The listing builds one solid part. Answer for the finished solid, in the listing's coordinates (mm). Face numbers are marked on the shaded views. Give positions to 0.01 mm unless a question says otherwise; leave off trailing zeros. Write each loop counter-clockwise with the first axis right and the second up, starting at its lowest first coordinate (ties: lowest second). Pieces come first, ordered by that corner, then holes.
```python
from build123d import *

# Parameters (mm, degrees)
SKETCH1_R           = 7
BOSS_EXTRUDE1_DEPTH = 1
SKETCH2_R           = 7
BOSS_EXTRUDE2_DEPTH = 4
SKETCH3_R           = 7.5
BOSS_EXTRUDE3_DEPTH = 1
SKETCH5_R           = 7
SKETCH7_R           = 7.5
BOSS_EXTRUDE4_DEPTH = 1
SKETCH8_R           = 7
BOSS_EXTRUDE5_DEPTH = 4
SKETCH9_R           = 7
BOSS_EXTRUDE6_DEPTH = 1
SKETCH11_R          = 6


with BuildPart() as part:
    # Sketch1 → Boss-Extrude1 (new body)
    with BuildSketch(Plane(origin=(0, 0, 0), x_dir=(1, 0, 0), z_dir=(0, 1, 0))):
        with Locations(Location((0, 0, 0), (0, 0, 270))):
            Circle(SKETCH1_R)
    extrude(amount=BOSS_EXTRUDE1_DEPTH)

    # Sketch2 → Boss-Extrude2 (add)
    with BuildSketch(Plane(origin=(0, 1, 0), x_dir=(1, 0, 0), z_dir=(0, 1, 0))):
        with Locations(Location((0, 0, 0), (0, 0, 270))):
            Circle(SKETCH2_R)
    extrude(amount=BOSS_EXTRUDE2_DEPTH)

    # Sketch3 → Boss-Extrude3 (add)
    with BuildSketch(Plane(origin=(0, 5, 0), x_dir=(1, 0, 0), z_dir=(0, 1, 0))):
        with Locations(Location((0, 0, 0), (0, 0, 270))):
            Circle(SKETCH3_R)
    extrude(amount=BOSS_EXTRUDE3_DEPTH)

    # Sweep1: sweep along a path in Sketch4
    with BuildLine(Plane.XY) as sweep1_path:
        ThreePointArc((0, 6), (6.443650814, 21.556349186), (22, 28))
    # Sketch5 → Sweep1 (sweep)
    with BuildSketch(Plane(origin=(0, 6, 0), x_dir=(1, 0, 0), z_dir=(0, 1, 0))):
        Circle(SKETCH5_R)
    sweep(path=sweep1_path.line)

    # Sketch7 → Boss-Extrude4 (add)
    with BuildSketch(Plane(origin=(22, 0, 0), x_dir=(0, 0, -1), z_dir=(1, 0, 0))):
        with Locations((0, 28)):
            Circle(SKETCH7_R)
    extrude(amount=BOSS_EXTRUDE4_DEPTH)

    # Sketch8 → Boss-Extrude5 (add)
    with BuildSketch(Plane(origin=(23, 0, 0), x_dir=(0, 0, -1), z_dir=(1, 0, 0))):
        with Locations((0, 28)):
            Circle(SKETCH8_R)
    extrude(amount=BOSS_EXTRUDE5_DEPTH)

    # Sketch9 → Boss-Extrude6 (add)
    with BuildSketch(Plane(origin=(27, 0, 0), x_dir=(0, 0, -1), z_dir=(1, 0, 0))):
        with Locations((0, 28)):
            Circle(SKETCH9_R)
    extrude(amount=BOSS_EXTRUDE6_DEPTH)

    # Cut-Sweep1: sweep along a path in Sketch10
    with BuildLine(Plane.XY) as cut_sweep1_path:
        Line((0, 0), (0, 6))
        ThreePointArc((0, 6), (6.443650814, 21.556349186), (22, 28))
        Line((22, 28), (28, 28))
    # Sketch11 → Cut-Sweep1 (sweep, cut)
    with BuildSketch(Plane.XZ):
        Circle(SKETCH11_R)
    sweep(path=cut_sweep1_path.line, mode=Mode.SUBTRACT)


solid = part.part
```
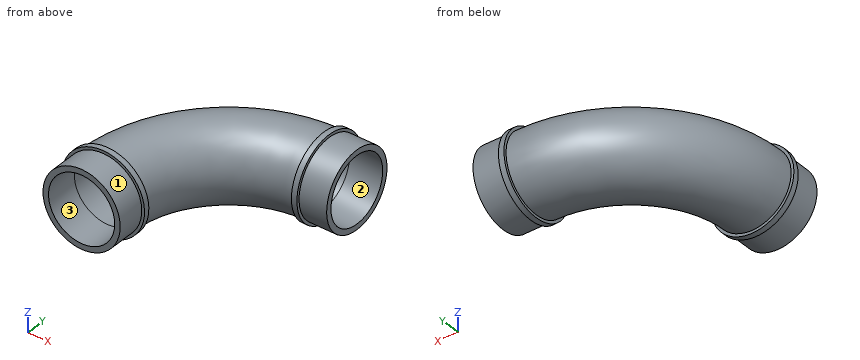
Item 1: A cutting plane is placed at A-A, the plane z = 0. Give the vertices of the cut face in (x, y), plus the area to 3 significant figures.
Conclusion:
outline: (-7.5, 5) - (-7, 5) - (-7, 0) - (-6, 0) - (-6, 6) arc R28 cw to (22, 34) - (28, 34) - (28, 35) - (23, 35) - (23, 35.5) - (22, 35.5) - (22, 35) arc R29 ccw to (-7, 6) - (-7.5, 6) - close; (6, 0) - (7, 0) - (7, 5) - (7.5, 5) - (7.5, 6) - (7, 6) arc R15 cw to (22, 21) - (22, 20.5) - (23, 20.5) - (23, 21) - (28, 21) - (28, 22) - (22, 22) arc R16 ccw to (6, 6) - close
area: 95.1 mm2
Item 2: Determine the mould class of the marked faces 1, 2 and 3 for opening direction X: pulls with the +X half, pulls with the -X half, needs draft (parallel to the pull), parting line crosses it, or undercut.
Conclusion:
face 1: parting line crosses it
face 2: needs draft
face 3: undercut
Item 3: A cutting plane is placed at B-B, the plane z = -5.5. Give the vertices of the cut face in (x, y), plus the area to 3 significant figures.
Conclusion:
outline: (-5.1, 5) - (-4.33, 5) - (-4.33, 0) - (-2.4, 0) - (-2.4, 6) arc R24.4 cw to (22, 30.4) - (28, 30.4) - (28, 32.33) - (23, 32.33) - (23, 33.1) - (22, 33.1) - (22, 32.33) arc R26.33 ccw to (-4.33, 6) - (-5.1, 6) - close; (2.4, 0) - (4.33, 0) - (4.33, 5) - (5.1, 5) - (5.1, 6) - (4.33, 6) arc R17.67 cw to (22, 23.67) - (22, 22.9) - (23, 22.9) - (23, 23.67) - (28, 23.67) - (28, 25.6) - (22, 25.6) arc R19.6 ccw to (2.4, 6) - close
area: 183 mm2
Item 4: Consider probe 1 along X at (y, z) = (4.3, 0); probe 2 along Y at (x, z) = (25, 0); probe 3 along Z at (x, y) = (3.5, 7). Determine where each line is inside the solid, lowest interval first.
Conclusion:
probe 1: x = -7 to -6, 6 to 7
probe 2: y = 21 to 22, 34 to 35
probe 3: z = -6.08 to -4.89, 4.89 to 6.08
Item 5: Each of these flat-tipped pins is pushed along its axis until it touches: P1, Ø8, axis at y = 12, z = 0, coming from the +X side; P2, Ø4.5, axis at y = 28, z = 2, coming from the +X side; P3, Ø4.5, axis at y = 28.5, z = 0, coming from the -X side. Where does it stop, or does it pass through?
Conclusion:
P1: stops at x = 10.82
P2: stops at x = 9.3
P3: stops at x = 1.24
